Geometry: final body of the model. Coordinates: model frame, mm. Face numbers are marked on the shaded views. A direction names the side the tool comes from. Coordinates: 2 decimals unless noted, no trailing zeros. Order: outer loops, then holes, each group sorted by start corner. A loop starts at its lowest first (then second) coordinate and runs counter-clockwise, first axis right, second up. Notation, with made-up numbers: (-7.5, 73) -> (42.5, 73) arc R31 ccw to (42.5, 105) -> close; hole circle Ø3 at (50.25, 11.25). An arc over 180 degrees is marked (long way). Answer in a Markdown table with one row per item. Add a question column.
1) Section query A-A on x = 0. Return the cut outline in (y, z).
2) Section query C-C on z = -5. Count the separate pieces of the cut face and the enclosed holes in it, then the cut area to 3 significant figures.
3) Ray query, line 1 (Y direction, x = 0, z = 6.25); line 2 (Y direction, x = 0, z = 11.7). Return the intervals inside material, ascending. Write a range as from..to.
4) Set-up query: the marked faces 1 and 2. Return all of +Z, -Z, +X, -X, +Y, -Y with unobstructed straight access to the full face (end or side cutting, diameter ignored); none if empty.
5) Contact query for flat-ended pins moving along their axis: P1, Ø19, axis at x = -2, y = 3, coming from the -Z side; P2, Ø12, axis at y = 31, z = -38, coming from the +X side; P3, Ø8, axis at x = 23, y = 49, coming from the +Z side. Output: stop coordinate, or through.
Autodesk Inventor part; units mm, degrees
ref_plane "YZ Plane" through (0, 0, 0) normal (1, 0, 0) x (0, 1, 0)
ref_plane "XZ Plane" through (0, 0, 0) normal (0, 1, 0) x (-1, 0, 0)
ref_plane "XY Plane" through (0, 0, 0) normal (0, 0, 1) x (1, 0, 0)
sketch "Sketch1" plane through (0, 0, 0) normal (0, 0, 1) x (1, 0, 0)
  point P0 (0, 0)
sketch "Sketch2" plane through (0, 0, 0) normal (0, 0, 1) x (1, 0, 0)
  circle A0 centre (0, 0) radius 75
  line L0 (-65.0875, -9.525) -> (-104.775, -39.6875) construction
  line L1 (-104.775, -39.6875) -> (-119.0625, -20.6375) construction
  line L2 (-119.0625, -20.6375) -> (-158.75, -15.875) construction
  line L3 (-158.75, -15.875) -> (-179.3875, -52.3875) construction
  spline S0 degree 4 poles (-65.0875, -9.525) (-104.775, -39.6875) (-119.0625, -20.6375) (-158.75, -15.875) (-179.3875, -52.3875) knots 1 1 1 1 1 2 2 2 2 2
  circle A1 centre (-65.0875, -9.525) radius 2.5
  dimension "d0" = 150
  dimension "d87" = 5
extrude "Extrusion1" add sketch "Sketch2" along normal blind 10 contours A0 | A1
hole "Hole1" at (0, 0, 0) direction (0, 0, 1) diameter 5 end through all
sketch "Sketch3" plane through (0, 0, 10) normal (0, 0, 1) x (1, 0, 0)
  point P0 (0, 0)
sketch "Sketch4" plane through (0, 0, 10) normal (0, 0, 1) x (1, 0, 0)
  point P0 (0, 0)
hole "Hole2" at (0, 0, 10) direction (0, 0, -1) diameter 20 end through all
chamfer "Chamfer1" distance 2 angle 45 1 edges at (0, 10, 10)
fillet "Fillet1" radius 2 1 edges at (-75, 0, 10)
fillet "Fillet2" radius 2 1 edges at (-75, 0, 0)
sketch "Sketch8" plane through (0, 0, 10) normal (0, 0, 1) x (1, 0, 0)
  circle A0 centre (0, 0) radius 10
  circle A1 centre (0, 0) radius 29.2721
extrude "Extrusion4" add sketch "Sketch8" along normal blind 5
chamfer "Chamfer2" distance 2 angle 45 1 edges at (-29.2721, 0, 15)
sketch "Sketch24" plane through (0, 0, 0) normal (1, 0, 0) x (0, 1, 0)
  line L0 (10, 0) -> (-10, 0)
  point P0 (0, 0)
sketch "Sketch25" plane through (0, 0, 0) normal (0, 0, 1) x (1, 0, 0)
  circle A0 centre (0, 0) radius 10
  circle A1 centre (0, 0) radius 73
  circle A2 centre (23.8125, -61.9125) radius 2.5
  circle A3 centre (51.5785, -41.7115) radius 2.5
  circle A4 centre (65.524, -10.334) radius 2.5
  circle A5 centre (61.9125, 23.8125) radius 2.5
  circle A6 centre (41.7115, 51.5785) radius 2.5
  circle A7 centre (10.334, 65.524) radius 2.5
  circle A8 centre (-23.8125, 61.9125) radius 2.5
  circle A9 centre (-51.5785, 41.7115) radius 2.5
  circle A10 centre (-65.524, 10.334) radius 2.5
  circle A11 centre (-61.9125, -23.8125) radius 2.5
  circle A12 centre (-41.7115, -51.5785) radius 2.5
  circle A13 centre (-10.334, -65.524) radius 2.5
  circle A14 centre (0, 0) radius 10
  circle A15 centre (0, 0) radius 10
  dimension "d104" = 5
  dimension "d107" = 360
sketch "Sketch26" plane through (0, 0, 0) normal (0, 0, -1) x (-1, 0, 0)
  point P0 (0, 0)
extrude "Extrusion6" add sketch "Sketch25" against normal blind 50 contours A3 | A4 | A5 | A6 | A7 | A8 | A9 | A10 | A11 | A12 | A13
sketch "Sketch28" plane through (0, 0, 0) normal (0, 0, -1) x (-1, 0, 0)
  circle A0 centre (-51.5785, -41.7115) radius 2.5
  circle A1 centre (65.524, 10.334) radius 2.5
  circle A2 centre (-51.5785, -41.7115) radius 2.5
  circle A3 centre (-10.334, 65.524) radius 2.5
  circle A4 centre (-65.524, -10.334) radius 2.5
  circle A5 centre (61.9125, -23.8125) radius 2.5
  circle A6 centre (51.5785, 41.7115) radius 2.5
  circle A7 centre (10.334, -65.524) radius 2.5
  circle A8 centre (-41.7115, 51.5785) radius 2.5
  circle A9 centre (-61.9125, 23.8125) radius 2.5
  circle A10 centre (41.7115, -51.5785) radius 2.5
  circle A11 centre (23.8125, 61.9125) radius 2.5
  circle A12 centre (0, 0) radius 10
  circle A13 centre (0, 0) radius 73
  circle A14 centre (65.524, 10.334) radius 2.5
  circle A15 centre (-51.5785, -41.7115) radius 2.5
  circle A16 centre (-10.334, 65.524) radius 2.5
  circle A17 centre (-65.524, -10.334) radius 2.5
  circle A18 centre (61.9125, -23.8125) radius 2.5
  circle A19 centre (51.5785, 41.7115) radius 2.5
  circle A20 centre (10.334, -65.524) radius 2.5
  circle A21 centre (-41.7115, 51.5785) radius 2.5
  circle A22 centre (-61.9125, 23.8125) radius 2.5
  circle A23 centre (41.7115, -51.5785) radius 2.5
  circle A24 centre (23.8125, 61.9125) radius 2.5
  circle A25 centre (0, 0) radius 10
  circle A26 centre (0, 0) radius 73
  circle A27 centre (65.524, 10.334) radius 2.5
  circle A28 centre (-51.5785, -41.7115) radius 2.5
  circle A29 centre (-10.334, 65.524) radius 2.5
  circle A30 centre (-65.524, -10.334) radius 2.5
  circle A31 centre (61.9125, -23.8125) radius 2.5
  circle A32 centre (51.5785, 41.7115) radius 2.5
  circle A33 centre (10.334, -65.524) radius 2.5
  circle A34 centre (-41.7115, 51.5785) radius 2.5
  circle A35 centre (-61.9125, 23.8125) radius 2.5
  circle A36 centre (41.7115, -51.5785) radius 2.5
  circle A37 centre (23.8125, 61.9125) radius 2.5
  circle A38 centre (0, 0) radius 10
  circle A39 centre (0, 0) radius 73
sketch "Sketch29" plane through (0, 0, 0) normal (0, 0, 1) x (1, 0, 0)
  circle A0 centre (23.8125, -61.9125) radius 2.5
  point P0 (0, 0)
  dimension "d111" = 5
extrude "Extrusion7" add sketch "Sketch29" against normal blind 50
properties part number "base"
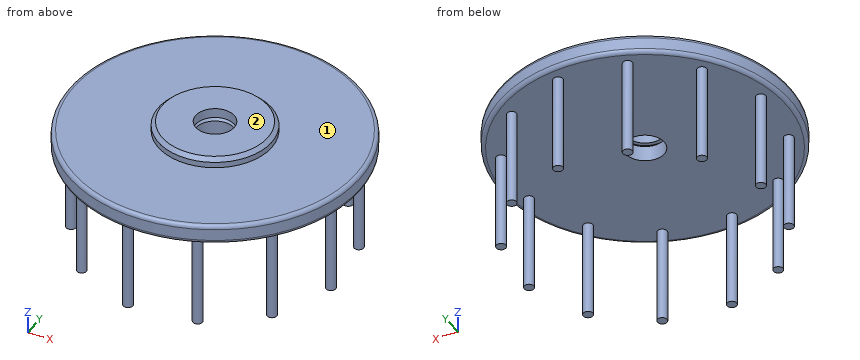
Result:
| question | item | result |
|---|---|---|
| 1 | outline | (-75, 2) arc R2 ccw to (-73, 0) -> (-10, 0) -> (-10, 8) -> (-12, 10) -> (-10, 10) -> (-10, 15) -> (-27.27, 15) -> (-29.27, 13) -> (-29.27, 10) -> (-73, 10) arc R2 ccw to (-75, 8) -> close; (10, 0) -> (73, 0) arc R2 ccw to (75, 2) -> (75, 8) arc R2 ccw to (73, 10) -> (29.27, 10) -> (29.27, 13) -> (27.27, 15) -> (10, 15) -> (10, 10) -> (12, 10) -> (10, 8) -> close |
| 2 | separate pieces | 12 |
| 2 | enclosed holes | 0 |
| 2 | area | 236 mm2 |
| 3 | line 1 | -75..-10, 10..75 |
| 3 | line 2 | -29.27..-10, 10..29.27 |
| 4 | face 1 | +Z |
| 4 | face 2 | +Z, +X, -X, +Y, -Y |
| 5 | P1 | z = 0 |
| 5 | P2 | x = 64.11 |
| 5 | P3 | z = 10 |
